Geometry: final body of the model. Coordinates: model frame, mm. Face numbers are marked on the shaded views. A direction names the side the tool comes from. Give positions to 0.01 mm unless a question says otherwise; leave off trailing zeros. Write each loop counter-clockwise with the first axis right and the second up, starting at its lowest first coordinate (ties: lowest second). Pieces come first, ordered by that corner, then holes. Notation, with made-up numbers: (-7.75, 68) - (40.25, 68) arc R21 cw to (40.25, 83) - close; hole circle Ø7 at (61, 76). An arc over 180 degrees is marked (long way). Use CSV: the item, a comma, the result in double quotes. Start each with the question number.
(1) Section A-A on y = -3.5. Output: boundary loops of the cut face in (x, z), and give its area (3 significant figures).
(2) Reachability of the marked faces 1, 2 and 3 from +Z, -Z, +X, -X, +Y, -Y: full face, straight path, thin tool, end or side. Return the list, or none.
(3) First-contact query: pin 1 Ø2.5 at (x, z) = (14.5, -18) entering from +Y; pin 2 Ø1.5 at (x, z) = (-18.5, -20) entering from +Y; pin 3 Ø2.5 at (y, z) = (-9.5, 21) entering from -X; pin 4 Ø22.5 at (x, z) = (-3, -6) entering from -Y. Flat tips, straight axial feed; report the tip coordinate or a pass-through.
(4) Draft query along Z for the marked faces 4, 5 and 6. Return one class per face: released by +Z, released by -Z, zero draft, split by the parting line, or undercut.
(5) Line query: probe 1 along X at (y, z) = (-23.75, 0); probe 2 along X at (y, z) = (2, 0); probe 3 along X at (y, z) = (-16.5, 11). Output: solid intervals per line, ascending. Write a range as [from, to].
(6) Section B-B on x = -2. Count the separate pieces of the cut face and the enclosed holes in it, and give its area (3 significant figures).
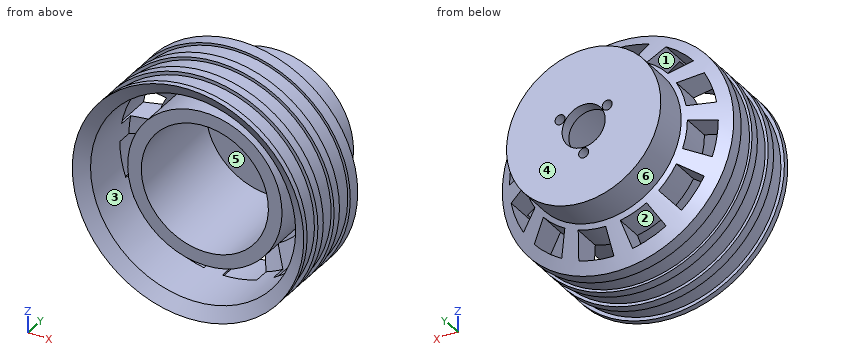
from build123d import *

# Parameters (mm, degrees)
SKETCH_2_R          = 4.75
SKETCH_2_R_2        = 1.1
CUT_EXTRUDE_1_DEPTH = 10
CUT_EXTRUDE_2_DEPTH = 17.5
SKETCH_9_R          = 26
SKETCH_9_R_2        = 24.954284739
CUT_EXTRUDE_4_DEPTH = 4
SKETCH_10_R         = 27.155658861
SKETCH_10_R_2       = 24.851094357
CUT_EXTRUDE_5_DEPTH = 4
SKETCH_11_R         = 26.970973613
SKETCH_11_R_2       = 24.736173034
CUT_EXTRUDE_6_DEPTH = 4


with BuildPart() as part:
    # 草图1 → 旋转1 (revolve)
    with BuildSketch(Plane.XY, mode=Mode.PRIVATE) as revolve_1_sk:
        Polygon((0, 2.5), (17, 2.5), (17, -24), (14, -24), (14, 0), (0, 0), align=None)
    revolve(revolve_1_sk.sketch.rotate(Axis((0, 0, 0), (0, 1, 0)), 90), axis=Axis((0, 0, 0), (0, 1, 0)))

    # 草图2 → 切除-拉伸1 (cut)
    with BuildSketch(Plane(origin=(0, 2.5, 0), x_dir=(1, 0, 0), z_dir=(0, 1, 0))):
        with Locations(Location((0, 0, 0), (0, 0, 270))):
            Circle(SKETCH_2_R)
        with Locations(Location((0, 6, 0), (0, 0, 270))):
            Circle(SKETCH_2_R_2)
        with Locations(Location((5.196152423, -3, 0), (0, 0, 270))):
            Circle(SKETCH_2_R_2)
        with Locations(Location((-5.196152423, -3, 0), (0, 0, 270))):
            Circle(SKETCH_2_R_2)
    extrude(amount=-CUT_EXTRUDE_1_DEPTH, mode=Mode.SUBTRACT)

    # 草图6 → 旋转3 (revolve)
    with BuildSketch(Plane(origin=(0, 0, 0), x_dir=(0, 0, -1), z_dir=(1, 0, 0)), mode=Mode.PRIVATE) as revolve_3_sk:
        Polygon((17, -11.545676787), (17, -5.056486478), (25.5, -10.238041423), (25.5, -30.238041423), (22.594733801, -28.353869151), (22.594733801, -14.08803646), align=None)
    revolve(revolve_3_sk.sketch.rotate(Axis((0, 0, 0), (0, -1, 0)), 180), axis=Axis((0, 0, 0), (0, -1, 0)))

    # 草图7 → 切除-拉伸2 (cut, symmetric)
    with BuildSketch(Plane(origin=(0, 0, 0), x_dir=(1, 0, 0), z_dir=(0, 1, 0))):
        with BuildLine():
            Line((0, 23), (0, 18))
            ThreePointArc((0, 18), (3.070781712, 17.736129783), (6.051531441, 16.95225552))
            Line((6.051531441, 16.95225552), (7.732512397, 21.661215387))
            ThreePointArc((7.732512397, 21.661215387), (3.923776632, 22.6628325), (0, 23))
        make_face()
        with BuildLine():
            Line((17.527159865, 14.892906603), (13.71690772, 11.655318211))
            ThreePointArc((13.71690772, 11.655318211), (11.527439863, 13.824548101), (9, 15.588457268))
            Line((9, 15.588457268), (11.5, 19.918584287))
            ThreePointArc((11.5, 19.918584287), (14.729506492, 17.664700351), (17.527159865, 14.892906603))
        make_face()
        with BuildLine():
            Line((22.625419, 4.134055522), (17.706849652, 3.2353478))
            ThreePointArc((17.706849652, 3.2353478), (16.895329813, 6.20868992), (15.588457268, 9))
            Line((15.588457268, 9), (19.918584287, 11.5))
            ThreePointArc((19.918584287, 11.5), (21.588476983, 7.933326009), (22.625419, 4.134055522))
        make_face()
        with BuildLine():
            Line((21.661215387, -7.732512397), (16.95225552, -6.051531441))
            ThreePointArc((16.95225552, -6.051531441), (17.736129783, -3.070781712), (18, 0))
            Line((18, 0), (23, 0))
            ThreePointArc((23, 0), (22.6628325, -3.923776632), (21.661215387, -7.732512397))
        make_face()
        with BuildLine():
            Line((14.892906603, -17.527159865), (11.655318211, -13.71690772))
            ThreePointArc((11.655318211, -13.71690772), (13.824548101, -11.527439863), (15.588457268, -9))
            Line((15.588457268, -9), (19.918584287, -11.5))
            ThreePointArc((19.918584287, -11.5), (17.664700351, -14.729506492), (14.892906603, -17.527159865))
        make_face()
        with BuildLine():
            Line((4.134055522, -22.625419), (3.2353478, -17.706849652))
            ThreePointArc((3.2353478, -17.706849652), (6.20868992, -16.895329813), (9, -15.588457268))
            Line((9, -15.588457268), (11.5, -19.918584287))
            ThreePointArc((11.5, -19.918584287), (7.933326009, -21.588476983), (4.134055522, -22.625419))
        make_face()
        with BuildLine():
            Line((-7.732512397, -21.661215387), (-6.051531441, -16.95225552))
            ThreePointArc((-6.051531441, -16.95225552), (-3.070781712, -17.736129783), (0, -18))
            Line((0, -18), (0, -23))
            ThreePointArc((0, -23), (-3.923776632, -22.6628325), (-7.732512397, -21.661215387))
        make_face()
        with BuildLine():
            Line((-17.527159865, -14.892906603), (-13.71690772, -11.655318211))
            ThreePointArc((-13.71690772, -11.655318211), (-11.527439863, -13.824548101), (-9, -15.588457268))
            Line((-9, -15.588457268), (-11.5, -19.918584287))
            ThreePointArc((-11.5, -19.918584287), (-14.729506492, -17.664700351), (-17.527159865, -14.892906603))
        make_face()
        with BuildLine():
            Line((-22.625419, -4.134055522), (-17.706849652, -3.2353478))
            ThreePointArc((-17.706849652, -3.2353478), (-16.895329813, -6.20868992), (-15.588457268, -9))
            Line((-15.588457268, -9), (-19.918584287, -11.5))
            ThreePointArc((-19.918584287, -11.5), (-21.588476983, -7.933326009), (-22.625419, -4.134055522))
        make_face()
        with BuildLine():
            Line((-21.661215387, 7.732512397), (-16.95225552, 6.051531441))
            ThreePointArc((-16.95225552, 6.051531441), (-17.736129783, 3.070781712), (-18, 0))
            Line((-18, 0), (-23, 0))
            ThreePointArc((-23, 0), (-22.6628325, 3.923776632), (-21.661215387, 7.732512397))
        make_face()
        with BuildLine():
            Line((-14.892906603, 17.527159865), (-11.655318211, 13.71690772))
            ThreePointArc((-11.655318211, 13.71690772), (-13.824548101, 11.527439863), (-15.588457268, 9))
            Line((-15.588457268, 9), (-19.918584287, 11.5))
            ThreePointArc((-19.918584287, 11.5), (-17.664700351, 14.729506492), (-14.892906603, 17.527159865))
        make_face()
        with BuildLine():
            Line((-4.134055522, 22.625419), (-3.2353478, 17.706849652))
            ThreePointArc((-3.2353478, 17.706849652), (-6.20868992, 16.895329813), (-9, 15.588457268))
            Line((-9, 15.588457268), (-11.5, 19.918584287))
            ThreePointArc((-11.5, 19.918584287), (-7.933326009, 21.588476983), (-4.134055522, 22.625419))
        make_face()
    extrude(amount=CUT_EXTRUDE_2_DEPTH, both=True, mode=Mode.SUBTRACT)

    # 草图9 → 切除-拉伸4 (cut)
    with BuildSketch(Plane(origin=(0, -13, 0), x_dir=(1, 0, 0), z_dir=(0, 1, 0))):
        Circle(SKETCH_9_R)
        with Locations(Location((0, 0, 0), (0, 0, 270))):
            Circle(SKETCH_9_R_2, mode=Mode.SUBTRACT)
    extrude(amount=-CUT_EXTRUDE_4_DEPTH, mode=Mode.SUBTRACT)

    # 草图10 → 切除-拉伸5 (cut)
    with BuildSketch(Plane(origin=(0, -19, 0), x_dir=(1, 0, 0), z_dir=(0, 1, 0))):
        Circle(SKETCH_10_R)
        with Locations(Location((0, 0, 0), (0, 0, 270))):
            Circle(SKETCH_10_R_2, mode=Mode.SUBTRACT)
    extrude(amount=-CUT_EXTRUDE_5_DEPTH, mode=Mode.SUBTRACT)

    # 草图11 → 切除-拉伸6 (cut)
    with BuildSketch(Plane(origin=(0, -25, 0), x_dir=(1, 0, 0), z_dir=(0, 1, 0))):
        Circle(SKETCH_11_R)
        with Locations(Location((0, 0, 0), (0, 0, 270))):
            Circle(SKETCH_11_R_2, mode=Mode.SUBTRACT)
    extrude(amount=-CUT_EXTRUDE_6_DEPTH, mode=Mode.SUBTRACT)


solid = part.part
Check values:
1,outline,"circle Ø34 at (0, 0); hole circle Ø28 at (0, 0)"
1,area,"292 mm²"
2,face 1,"+Y"
2,face 2,"+Y, -Y"
2,face 3,"-Y"
3,pin 1,"stops at y = -8.71"
3,pin 2,"passes through"
3,pin 3,"stops at x = -15.83"
3,pin 4,"stops at y = -24"
4,face 4,"zero draft"
4,face 5,"undercut"
4,face 6,"split by the parting line"
5,probe 1,"x = [-25.5, -22.59], [-17, -14], [14, 17], [22.59, 25.5]"
5,probe 2,"x = [-17, -4.75], [4.75, 17]"
5,probe 3,"x = [-22.4, -20.2], [-12.96, -8.66], [8.66, 12.96], [19.74, 22.4]"
6,separate pieces,"3"
6,enclosed holes,"0"
6,area,"346 mm²"
